The model under review builds one solid part; all positions refer to its coordinate system, in mm. A direction names the side the tool comes from. Round coordinates to 2 decimals unless told otherwise and drop trailing zeros. Write each loop counter-clockwise with the first axis right and the second up, starting at its lowest first coordinate (ties: lowest second). Pieces come first, ordered by that corner, then holes. Notation, with made-up numbers: (-8.75, 82) -> (43.25, 82) arc R12 ccw to (43.25, 94) -> close; hole circle Ø11 at (17, 65). An arc over 180 degrees is marked (long way). Answer as a JSON object with one key per item and string values. Group by question number.
1) Insertion check: pin 1 Ø1.8 at (x, z) = (-21.5, 3.5) entering from -Y; pin 2 Ø1.5 at (y, z) = (6.5, 4) entering from +X; pin 3 Ø1.8 at (y, z) = (1.5, 3) entering from -X. Each pin has a flat end and moves straight along its axis. Give the tip position at first contact, or say it passes through.
2) We need section C-C, the plane x = -17.5. Write out the cut boundary in (y, z), then the cut area to 3 significant figures.
3) Machinability: for faces 1 (the flat face through (-20, 10, 3)), 2 (the flat face through (-21, -10, 3)), 3 (the flat face through (5, 6, 3)), which of the approach directions +Z, -Z, +X, -X, +Y, -Y give a long, thin tool a straight path to every point of the face, cutting with its end or side? Answer none if there is none.
4) We need section B-B, the plane z = 3.3. Count the separate pieces of the cut face and the enclosed holes in it, then the cut area to 3 significant figures.
5) To check wall thickness, follow probe 1 along X at (y, z) = (0, 4.7); probe 2 along X at (y, z) = (-1.25, 4.8); probe 3 along Y at (x, z) = (60, 1.35). State the ranges of each line that lie inside material, in increasing order. Write a range as [from, to].
6) We need section A-A, the plane y = 4.75. Write out the cut boundary in (x, z), then the cut area to 3 significant figures.
7) Mouldability with a two-part tool opening along Y and no side actions: class faces 4 (the flat face through (-42.98, -8.948, 2.958)), 5 (the flat face through (42.99, 8.94, 2.96)), 6 (the flat face through (-6, 0, 3)) as pulls with the +Y half, pulls with the -Y half, needs draft (parallel to the pull), parting line crosses it, or undercut.
Solid Edge part; units mm, degrees
sketch "Sketch1" plane through (0, 0, 0) normal (0, 0, 1) x (1, 0, 0)
  line L0 (-15.95, 10) -> (-25, 10)
  line L1 (-25, 10) -> (-60.4638, 7.9246)
  line L2 (-60.4638, -7.9246) -> (-25, -10)
  line L3 (-25, -10) -> (-15.95, -10)
  arc A0 (-15.95, -10) -> (-14.75, -11.2) centre (-15.95, -11.2) cw
  line L4 (-14.75, -11.2) -> (-14.75, -11.3)
  arc A1 (-14.75, -11.3) -> (-13.55, -12.5) centre (-13.55, -11.3) ccw
  line L5 (-13.55, -12.5) -> (24.05, -12.5)
  arc A2 (25.25, -11.3) -> (24.05, -12.5) centre (24.05, -11.3) cw
  line L6 (25.25, -11.3) -> (25.25, -11.1172)
  arc A3 (25.25, -11.1172) -> (26.3799, -9.9192) centre (26.45, -11.1172) cw
  line L7 (26.3799, -9.9192) -> (60.4639, -7.9238)
  line L8 (26.3795, 9.9189) -> (60.069, 7.9371)
  arc A4 (25.25, 11.1168) -> (26.3795, 9.9189) centre (26.45, 11.1168) ccw
  line L9 (25.25, 11.1168) -> (25.25, 11.295)
  arc A5 (24.045, 12.5) -> (25.25, 11.295) centre (24.045, 11.295) cw
  line L10 (24.045, 12.5) -> (-13.55, 12.5)
  arc A6 (-14.75, 11.3) -> (-13.55, 12.5) centre (-13.55, 11.3) cw
  line L11 (-14.75, 11.3) -> (-14.75, 11.2)
  arc A7 (-15.95, 10) -> (-14.75, 11.2) centre (-15.95, 11.2) ccw
  arc A8 (-60.4638, -7.9246) -> (-60.4638, 7.9246) centre (-60, 0) cw
  arc A9 (60.069, 7.9371) -> (60.4639, -7.9238) centre (60, 0) cw
extrude "Protrusion1" add sketch "Sketch1" along normal blind 6
sketch "Sketch2" plane through (0, 0, 0) normal (0, 0, 1) x (1, 0, 0)
  circle A0 centre (-60, 0) radius 1.56
  circle A1 centre (60, 0) radius 1.56
extrude "ExtrudedCutout_1" cut sketch "Sketch2" along normal blind 17.9181
sketch "Sketch3" plane through (0, 0, 0) normal (0, 0, 1) x (1, 0, 0)
  line L0 (-6, 6) -> (16.5, 6)
  line L1 (16.5, 6) -> (16.5, -6)
  line L2 (16.5, -6) -> (-6, -6)
  line L3 (-6, -6) -> (-6, 0)
  line L4 (-6, 0) -> (-6, 6)
  arc A0 (-8, 1) -> (-8, -1) centre (-8, 0) cw
  line L5 (-10, -1) -> (-8, -1)
  arc A1 (-10, -1) -> (-10, 1) centre (-10, 0) cw
  line L6 (-10, 1) -> (-8, 1)
  arc A2 (20.5, -1) -> (20.5, 1) centre (20.5, 0) ccw
  line L7 (20.5, 1) -> (18.5, 1)
  arc A3 (18.5, 1) -> (18.5, -1) centre (18.5, 0) ccw
  line L8 (20.5, -1) -> (18.5, -1)
extrude "ExtrudedCutout_2" cut sketch "Sketch3" along normal blind 36.5435
Here are the results:
{
 "1": {"pin 1": "stops at y = -10", "pin 2": "stops at x = 65.47", "pin 3": "stops at x = -67.92"},
 "2": {"outline": "(-10, 0) -> (10, 0) -> (10, 6) -> (-10, 6) -> close", "area": "120 mm^2"},
 "3": {"face 1": "+Z, -Z, -X, +Y", "face 2": "+Z, -Z, -X, -Y", "face 3": "+Z, -Z"},
 "4": {"separate pieces": "1", "enclosed holes": "5", "area": "2,350 mm^2"},
 "5": {"probe 1": "x = [-67.94, -61.56], [-58.44, -11], [-7, -6], [16.5, 17.5], [21.5, 58.44], [61.56, 67.94]", "probe 2": "x = [-67.84, -60.93], [-59.07, -6], [16.5, 59.07], [60.93, 67.84]", "probe 3": "y = [-7.95, -1.56], [1.56, 7.94]"},
 "6": {"outline": "(-66.36, 0) -> (-6, 0) -> (-6, 6) -> (-66.36, 6) -> close; (16.5, 0) -> (66.36, 0) -> (66.36, 6) -> (16.5, 6) -> close", "area": "661 mm^2"},
 "7": {"face 4": "pulls with the -Y half", "face 5": "pulls with the +Y half", "face 6": "undercut"}
}
